```python
from build123d import *

# Parameters (mm, degrees)
F0_R       = 11.176
F1_DEPTH   = 7.62
F2_SIZE2   = 2.1997045256
F2_SIZE    = 3.81
F2_2_SIZE2 = 2.1997045256
F2_2_SIZE  = 3.81
F3_SIZE2   = 2.1997045256
F3_SIZE    = 3.81
F4_SIZE    = 2.54


# Not quite as in the source:
# - a feature names something its author has since deleted; it is built from what else it names


with BuildPart() as f1:
    # F0 (on Top) → F1 (new body)
    with BuildSketch(Plane.XY):
        with BuildLine():
            ThreePointArc((9.7057271537, 23.5283748909), (-0.0208649872, 15.4470615517), (-9.6943160077, 23.5919105566))
            Line((-9.6943160077, 23.5919105566), (-19.3886320155, 27.4654462223))
            Line((-19.3886320155, 27.4654462223), (-28.8233609262, 31.2352592656))
            Line((-28.8233609262, 31.2352592656), (-51.1347862104, 30.8821881406))
            Line((-51.1347862104, 30.8821881406), (-41.4352900784, 9.4122263494))
            Line((-41.4352900784, 9.4122263494), (-33.4914395336, 3.0781251091))
            Line((-33.4914395336, 3.0781251091), (-25.3390191684, -3.4222811682))
            ThreePointArc((-25.3390191684, -3.4222811682), (-13.4326493579, -7.7553437227), (-15.6332920147, -20.2330937227))
            Line((-15.6332920147, -20.2330937227), (-14.0799852263, -30.5435))
            Line((-14.0799852263, -30.5435), (-12.5664179144, -40.5901269958))
            Line((-12.5664179144, -40.5901269958), (-0.1099852263, -59.7535))
            Line((-0.1099852263, -59.7535), (12.5802445818, -40.4983495315))
            Line((12.5802445818, -40.4983495315), (14.0938118937, -30.4517225357))
            Line((14.0938118937, -30.4517225357), (15.6402053484, -20.1872049906))
            ThreePointArc((15.6402053484, -20.1872049906), (13.4326493579, -7.7553437227), (25.3027350274, -3.4512126568))
            Line((25.3027350274, -3.4512126568), (33.4188712518, 3.0202621318))
            Line((33.4188712518, 3.0202621318), (41.3627217965, 9.3543633721))
            Line((41.3627217965, 9.3543633721), (51.6930563519, 29.845))
            Line((51.6930563519, 29.845), (28.868872164, 31.0509006464))
            Line((28.868872164, 31.0509006464), (19.4114543073, 27.3383748909))
            Line((19.4114543073, 27.3383748909), (9.7057271537, 23.5283748909))
        make_face()
        with Locations((0, -30.48)):
            Circle(F0_R, mode=Mode.SUBTRACT)
        Circle(F0_R, mode=Mode.SUBTRACT)
        with Locations((-26.3964543073, 15.24)):
            Circle(F0_R, mode=Mode.SUBTRACT)
        with Locations((26.3964543073, 15.24)):
            Circle(F0_R, mode=Mode.SUBTRACT)
    extrude(amount=F1_DEPTH)

    # F2
    f2_edges = [f1.edges().sort_by_distance(p)[0] for p in [
        (-46.285038, 20.147207, 7.62),
        (-39.979074, 31.058724, 7.62),
        (40.280964, 30.44795, 7.62),
        (46.527889, 19.599682, 7.62),
        (6.23513, -50.125925, 7.62),
        (-6.338202, -50.171813, 7.62),
    ]]
    f2_side = f1.faces().sort_by_distance((19.789019, 26.011541, 7.62))[0]
    chamfer(f2_edges, length=F2_SIZE, length2=F2_SIZE2, reference=f2_side)

    # F2#2
    f2_2_edges = [f1.edges().sort_by_distance(p)[0] for p in [
        (-46.285038, 20.147207, 0),
        (46.527889, 19.599682, 0),
        (-39.979074, 31.058724, 0),
    ]]
    f2_2_side = f1.faces().sort_by_distance((19.789019, 26.011541, 0))[0]
    chamfer(f2_2_edges, length=F2_2_SIZE, length2=F2_2_SIZE2, reference=f2_2_side)

    # F3
    f3_edges = [f1.edges().sort_by_distance(p)[0] for p in [
        (-6.338202, -50.171813, 0),
        (6.23513, -50.125925, 0),
        (38.202915, 30.557743, 0),
    ]]
    f3_side = f1.faces().sort_by_distance((-15.154017, 24.375179, 0))[0]
    chamfer(f3_edges, length=F3_SIZE, length2=F3_SIZE2, reference=f3_side)

    # F4
    f4_edges = [f1.edges().sort_by_distance(p)[0] for p in [
        (-0.020865, 15.447062, 7.62),
        (13.432649, -7.755344, 7.62),
        (-13.432649, -7.755344, 7.62),
        (-13.432649, -7.755344, 0),
        (-0.020865, 15.447062, 0),
        (13.432649, -7.755344, 0),
    ]]
    chamfer(f4_edges, length=F4_SIZE)


solid = f1.part
```
Could you check a few things on this model? Use its own coordinates, in mm. Coordinates: 2 decimals unless noted, no trailing zeros. Loops run counter-clockwise (first coordinate to the right, second up) from the corner with the lowest first, then second, coordinate; pieces in that order, holes last.
1) Thinking about a two-plate mould opening in X: for faces 1 (the face through (-7.165, -45.453, 6.505)), 2 (the face through (13.222, -7.878, 5.203)), 3 (the face through (6.813, -45.836, 6.505)), which applies, released by +X, released by -X, zero draft, split by the parting line, or undercut?
Reported:
face 1: released by -X
face 2: undercut
face 3: released by +X
2) Will these pins go through, and if not, where does the flat tip stop? pin 1 Ø2 at (y, z) = (14.5, 3) entering from -X; pin 2 Ø18 at (x, y) = (0, 0) entering from +Z; pin 3 Ø1.5 at (y, z) = (0.5, 6) entering from +X; pin 4 Ø2 at (x, z) = (30.5, 1) entering from +Y.
Reported:
pin 1: stops at x = -44.19
pin 2: passes through
pin 3: stops at x = 31.2
pin 4: stops at y = 30.62
3) Please list where these lines run through material, in increasing order: line 1 along Y through (x, z) = (-2.5, 3.75); line 2 along Y through (x, z) = (1, 2.5); line 3 along X through (y, z) = (-13, 4.25).
Reported:
line 1: y = -56.08 to -41.37, -19.59 to -10.89, 10.89 to 15.77
line 2: y = -58.07 to -41.61, -19.35 to -11.13, 11.13 to 15.46
line 3: x = -12.12 to 12.12
4) Imagine slicing it at A-A (y = -25). List the corners of the cut face in (x, z) for me.
Reported:
outline: (-14.92, 0) - (-9.74, 0) - (-9.74, 7.62) - (-14.92, 7.62) - close; (9.74, 0) - (14.92, 0) - (14.92, 7.62) - (9.74, 7.62) - close
